Here's how the part is built. I have some questions about the finished solid (model axes, mm). A direction names the side the tool comes from. Give positions to 0.01 mm unless a question says otherwise; leave off trailing zeros. Loops run counter-clockwise (first coordinate to the right, second up) from the corner with the lowest first, then second, coordinate; pieces in that order, holes last.
Q1. Suppose I cut it at A-A (x = 0). List the corners of the cut face in (y, z) for me (3 decimals).
Q2. Suppose I cut it at C-C (x = -12). List the corners of the cut face in (y, z) for me, and give its area (3 significant figures).
Q3. I'm going to push flat-ended pins straight in: P1, Ø1.5, axis at x = 12, z = 1.5, coming from the -Y side; P2, Ø1, axis at x = 14.5, z = 5, coming from the -Y side; P3, Ø4, axis at x = 0, y = 0, coming from the -Z side; P4, Ø2, axis at y = -12, z = 2.5, coming from the -X side. Where does each tip first touch, or does it pass through?
Q4. Thinking about a two-plate mould opening in X: for faces 1 (the face through (12.049, -14.854, 3.219)), 2 (the face through (-19.875, 4.231, 3.131)), 3 (the face through (0, -4, 0)), 4 (the face through (17.85, 6.87, 3.22)), which applies, pulls with the +X half, pulls with the -X half, needs draft (parallel to the pull), parting line crosses it, or undercut?
Q5. For faces 5 (the face through (-2.977, -18.893, 3.219)), 6 (the face through (2.13, 20.21, 3.13)), 7 (the face through (1, 19.06, 3.22)), 8 (the face through (-18.89, -3.01, 3.22)), 9 (the face through (18.89, 3.01, 3.22)), which set-ups out of +Z, -Z, +X, -X, +Y, -Y let a thin tool reach every point of the face, with its end or its side?
Q6. I need wall thicknesses on probe 1 along Y at (x, z) = (0, 3.5) (3 decimals); probe 2 along X at (y, z) = (-17, 3.75); probe 3 along Y at (x, z) = (18, 5.5). Which ranges of each line are inside material? Lowest first, please.
Q7. Suppose I cut it at B-B (y = 2). List the corners of the cut face in (x, z) for me, and give its area (3 significant figures).
```python
from build123d import *

# Parameters (mm, degrees)
SKETCH1_R           = 20.32
OUTER_CIRCLE_DEPTH  = 6.35
TOOTH_CUT_DEPTH     = 30.430040775
TEETH_PATTERN_COUNT = 30
SKETCH3_R           = 3.175
CUT_EXTRUDE1_DEPTH  = 30.382561533


with BuildPart() as part:
    # Sketch1 → Outer Circle (new body)
    with BuildSketch(Plane.XY):
        Circle(SKETCH1_R)
    extrude(amount=OUTER_CIRCLE_DEPTH)

    # Sketch2 → Tooth Cut (cut, through all)
    with BuildSketch(Plane.XY.offset(6.35)):
        with BuildLine():
            ThreePointArc((-0.743845606, 17.764433391), (0, 17.78), (0.743845606, 17.764433391))
            ThreePointArc((0.743845606, 17.764433391), (1.009950749, 19.081439594), (1.671040922, 20.251173355))
            ThreePointArc((1.671040922, 20.251173355), (0, 20.32), (-1.671040922, 20.251173355))
            ThreePointArc((-1.671040922, 20.251173355), (-1.009950749, 19.081439594), (-0.743845606, 17.764433391))
        make_face()
    tooth_cut = extrude(amount=-TOOTH_CUT_DEPTH, mode=Mode.SUBTRACT)

    # Teeth Pattern: Tooth Cut ×30 about axis
    teeth_pattern_axis = Axis((0, 0, 0), (0, 0, 1))
    for i in range(1, TEETH_PATTERN_COUNT):
        add(tooth_cut.rotate(teeth_pattern_axis, i * 360 / TEETH_PATTERN_COUNT), mode=Mode.SUBTRACT)

    # Sketch3 → Cut-Extrude1 (cut, through all)
    with BuildSketch(Plane.XY.offset(6.35)):
        Circle(SKETCH3_R)
    extrude(amount=-CUT_EXTRUDE1_DEPTH, mode=Mode.SUBTRACT)


solid = part.part
```
Solutions:
1. outline: (-17.78, 0) - (-3.175, 0) - (-3.175, 6.35) - (-17.78, 6.35) - close; (3.175, 0) - (17.78, 0) - (17.78, 6.35) - (3.175, 6.35) - close
2. outline: (-14.82, 0) - (14.82, 0) - (14.82, 6.35) - (-14.82, 6.35) - close
2. area: 188 mm2
3. P1: stops at y = -15.23
3. P2: stops at y = -12.07
3. P3: passes through
3. P4: stops at x = -16.7
4. face 1: undercut
4. face 2: pulls with the -X half
4. face 3: needs draft
4. face 4: pulls with the +X half
5. face 5: +Z, -Z
5. face 6: +Z, -Z, +X, +Y
5. face 7: +Z, -Z, +Y
5. face 8: +Z, -Z, -X
5. face 9: +Z, -Z, +X
6. probe 1: y = -17.78 to -3.175, 3.175 to 17.78
6. probe 2: x = -10.55 to -8.66, -6.7 to 6.7, 8.66 to 10.55
6. probe 3: y = -8.72 to -6.99, -4.93 to -2.68, -1.13 to 1.13, 2.68 to 4.93, 6.99 to 8.72
7. outline: (-17.67, 0) - (-2.47, 0) - (-2.47, 6.35) - (-17.67, 6.35) - close; (2.47, 0) - (17.67, 0) - (17.67, 6.35) - (2.47, 6.35) - close
7. area: 193 mm2
